```python
from build123d import *

# Parameters (mm, degrees)
BOSS_EXTRUDE2_DEPTH = 6.35
FILLET1_R           = 12.7
FILLET2_R           = 12.7
FILLET3_R           = 12.7
FILLET4_R           = 12.7


with BuildPart() as part:
    # Sketch6 → Boss-Extrude2 (new body)
    with BuildSketch(Plane.XY):
        Polygon((-203.2, -355.396143874), (0, -507.797500764), (203.2, -355.396143874), (218.440086841, -375.716078743), (15.240086841, -528.117435634), (15.240086841, -629.717435634), (-15.240086841, -629.717435634), (-15.240086841, -528.117435634), (-218.440086841, -375.716078743), align=None)
    extrude(amount=BOSS_EXTRUDE2_DEPTH)

    # Fillet1
    fillet1_edges = [part.edges().sort_by_distance(p)[0] for p in [
        (203.2, -355.396143874, 3.175),
    ]]
    fillet(fillet1_edges, radius=FILLET1_R)

    # Fillet2
    fillet2_edges = [part.edges().sort_by_distance(p)[0] for p in [
        (218.440086841, -375.716078743, 3.175),
    ]]
    fillet(fillet2_edges, radius=FILLET2_R - 0.0001)  # a hair under: the kernel refuses the full size

    # Fillet3
    fillet3_edges = [part.edges().sort_by_distance(p)[0] for p in [
        (-203.2, -355.396143874, 3.175),
    ]]
    fillet(fillet3_edges, radius=FILLET3_R)

    # Fillet4
    fillet4_edges = [part.edges().sort_by_distance(p)[0] for p in [
        (-218.440086841, -375.716078743, 3.175),
    ]]
    fillet(fillet4_edges, radius=FILLET4_R - 0.0001)  # a hair under: the kernel refuses the full size


solid = part.part
```
Model file for the job. Use its own axes, mm. Coordinates: 2 decimals unless noted, no trailing zeros. Loops run counter-clockwise (first coordinate to the right, second up) from the corner with the lowest first, then second, coordinate; pieces in that order, holes last. Notation, with made-up numbers: (11.5, 3) - (35.5, 3) arc R23 cw to (35.5, 24) - close; hole circle Ø6 at (4.25, 79.25). An arc over 180 degrees is marked (long way). Write item = value, one per line. Start each with the question number.
Item 1: Saw through at D-D, the plane x = 100. List the corners of the cut face in (y, z), then the cut area to 3 significant figures.
Item 2: Saw through at A-A, the plane y = -414.5. List the corners of the cut face in (x, z), then the cut area to 3 significant figures.
Item 3: Drop flat-ended pins along their axis: pin 1 Ø1 at (x, z) = (-169, 1) entering from -Y; pin 2 Ø2 at (y, z) = (-413, 4.5) entering from +X; pin 3 Ø2 at (x, z) = (119.5, 2) entering from +Y. Give the stop position or say it passes through.
Item 4: Wall check: probe 1 along X at (y, z) = (-606, 0.5); probe 2 along X at (y, z) = (-421, 4.25); probe 3 along X at (y, z) = (-378, 3.25). Give the ranges that are in metal, low to high. Write a range as [from, to].
Item 5: Pull direction X, two halves, no side cores. Call faces 1 (the face through (-110.41, -456.74, 3.13)), 2 (the face through (-97.871, -434.393, 3.131)), 3 (the face through (33, -484, 0)), 4 (the face through (95.17, -436.42, 3.13)): +X half, -X half, draft (parallel to the pull), parting line (faces both ways), or undercut.
Item 6: Saw through at C-C, the plane y = -580.5. List the corners of the cut face in (x, z).
Answers:
q1.outline = (-464.55, 0) - (-432.8, 0) - (-432.8, 6.35) - (-464.55, 6.35) - close
q1.area = 202 mm2
q2.outline = (-166.73, 0) - (-124.4, 0) - (-124.4, 6.35) - (-166.73, 6.35) - close; (124.4, 0) - (166.73, 0) - (166.73, 6.35) - (124.4, 6.35) - close
q2.area = 538 mm2
q3.pin_1 = -413.17
q3.pin_2 = 170.06
q3.pin_3 = -417.42
q4.probe_1 = [-15.24, 15.24]
q4.probe_2 = [-158.06, -115.73], [115.73, 158.06]
q4.probe_3 = [-212.41, -173.06], [173.06, 212.41]
q5.face_1 = -X half
q5.face_2 = undercut
q5.face_3 = draft
q5.face_4 = undercut
q6.outline = (-15.24, 0) - (15.24, 0) - (15.24, 6.35) - (-15.24, 6.35) - close
